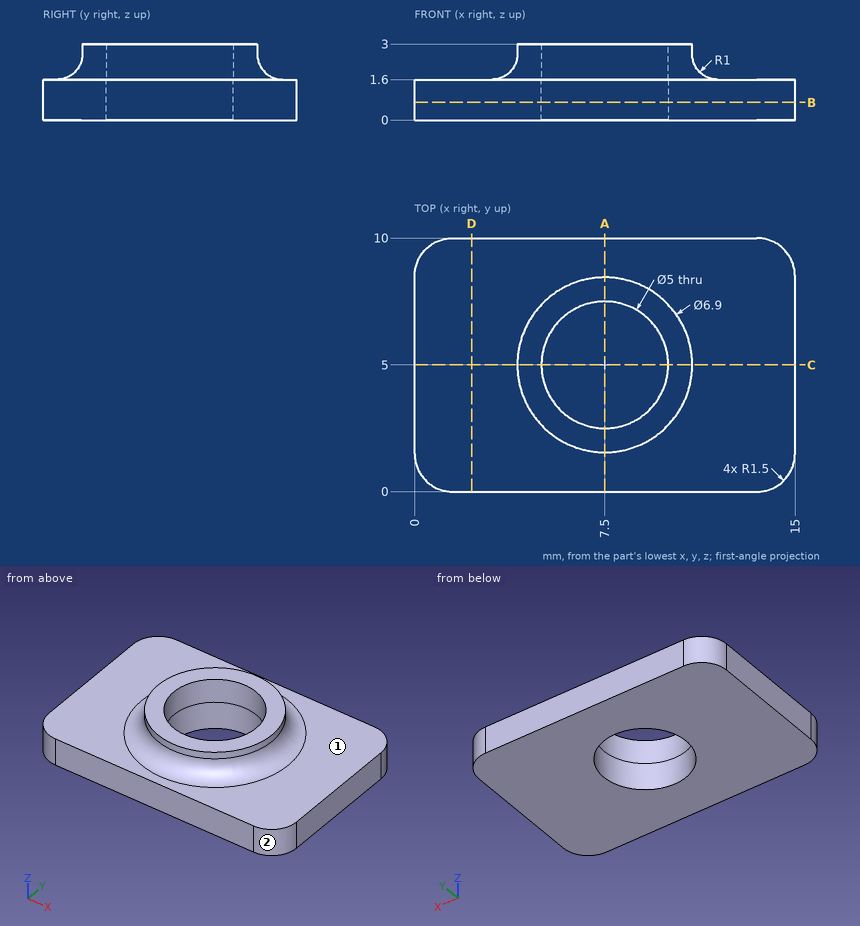
Could you check a few things on this drawing? It's one solid part, dimensions in mm from its lowest x, y, z. A direction names the side the tool comes from. Coordinates: 2 decimals unless noted, no trailing zeros. Order: outer loops, then holes, each group sorted by start corner. A loop starts at its lowest first (then second) coordinate and runs counter-clockwise, first axis right, second up. Notation, with made-up numbers: M 41.5,-25 L 77.5,-25 A31 ccw 77.5,7 Z; hole C -12,53.25 d5. An arc over 180 degrees is marked long. Answer as a JSON object with one key per item and string values. Group by question number.
(1) I need wall thicknesses on probe 1 along Y at (x, z) = (7.5, 0.55); probe 2 along Y at (x, z) = (7.5, 2.7); probe 3 along X at (y, z) = (4.75, 1.55). Which ranges of each line are inside material? Lowest first, please.
(2) Which directions (+Z, -Z, +X, -X, +Y, -Y) give clear straight access to the entire face, cutting with the end or side of a thin tool? Please do the marked faces 1 and 2.
(3) Suppose I cut it at C-C, the plane y = 5. Please give me the cut outline in (x, z).
(4) Suppose I cut it at D-D, the plane x = 2.25. Please give me the cut outline in (y, z), then the cut area to 3 significant figures.
(5) Suppose I cut it at A-A, the plane x = 7.5. Please give me the cut outline in (y, z).
(6) Suppose I cut it at B-B, the plane z = 0.7. Please give me the cut outline in (x, y), then the cut area to 3 significant figures.
Values found:
{
 "1": {"probe 1": "y = 0 to 2.5, 7.5 to 10", "probe 2": "y = 1.55 to 2.5, 7.5 to 8.45", "probe 3": "x = 0 to 5.01, 9.99 to 15"},
 "2": {"face 1": "+Z", "face 2": "+Z, -Z, +X, -Y"},
 "3": {"outline": "M 0,0 L 5,0 L 5,3 L 4.05,3 L 4.05,2.6 A1 cw 3.05,1.6 L 0,1.6 Z; M 10,0 L 15,0 L 15,1.6 L 11.95,1.6 A1 cw 10.95,2.6 L 10.95,3 L 10,3 Z"},
 "4": {"outline": "M 0,0 L 10,0 L 10,1.6 L 0,1.6 Z", "area": "16.0 mm^2"},
 "5": {"outline": "M 0,0 L 2.5,0 L 2.5,3 L 1.55,3 L 1.55,2.6 A1 cw 0.55,1.6 L 0,1.6 Z; M 7.5,0 L 10,0 L 10,1.6 L 9.45,1.6 A1 cw 8.45,2.6 L 8.45,3 L 7.5,3 Z"},
 "6": {"outline": "M 0,1.5 A1.5 ccw 1.5,0 L 13.5,0 A1.5 ccw 15,1.5 L 15,8.5 A1.5 ccw 13.5,10 L 1.5,10 A1.5 ccw 0,8.5 Z; hole C 7.5,5 d5", "area": "128 mm^2"}
}
